The model under review builds one solid part; all positions refer to its coordinate system, in mm. A direction names the side the tool comes from. Coordinates: 2 decimals unless noted, no trailing zeros. Write each loop counter-clockwise with the first axis right and the second up, starting at its lowest first coordinate (ties: lowest second). Pieces come first, ordered by that corner, then holes. Notation, with made-up numbers: (51, -33.5) - (109, -33.5) arc R20 ccw to (109, -17.5) - close; hole circle Ø10 at (28, -27). An arc over 180 degrees is marked (long way). Put each result on its own line as item: value.
Autodesk Inventor part; units mm, degrees
ref_plane "YZ Plane" through (0, 0, 0) normal (1, 0, 0) x (0, 1, 0)
ref_plane "XZ Plane" through (0, 0, 0) normal (0, 1, 0) x (-1, 0, 0)
ref_plane "XY Plane" through (0, 0, 0) normal (0, 0, 1) x (1, 0, 0)
sketch "Sketch1" plane through (0, 0, 0) normal (0, 0, 1) x (1, 0, 0)
  line L0 (0, 0) -> (50.8, 0)
  line L1 (50.8, 0) -> (50.8, 50.8)
  line L2 (50.8, 50.8) -> (0, 50.8)
  line L3 (0, 50.8) -> (0, 0)
  dimension "d0" = 50.8
  dimension "d1" = 50.8
extrude "Extrusion1" add sketch "Sketch1" along normal blind 50.8
sketch "Sketch2" plane through (0, 0, 50.8) normal (0, 0, 1) x (1, 0, 0)
  point P0 (0, 0)
sketch "Sketch3" plane through (0, 0, 50.8) normal (0, 0, 1) x (1, 0, 0)
  circle A0 centre (25.4, 25.4) radius 12.7
  line L0 (0, 50.8) -> (0, 0)
  line L1 (50.8, 50.8) -> (0, 50.8)
  dimension "d4" = 25.4
  dimension "d5" = 25.4
  dimension "d6" = 25.4
extrude "Extrusion2" cut sketch "Sketch3" against normal blind 50.8
sketch "Sketch4" plane through (50.8, 0, 0) normal (1, 0, 0) x (0, 0, -1)
  circle A0 centre (-25.4, 25.4) radius 12.7
  line L0 (-50.8, 0) -> (-50.8, 50.8)
  line L1 (0, 0) -> (0, 50.8)
  line L2 (0, 0) -> (-50.8, 0)
  dimension "d9" = 25.4
  dimension "d10" = 25.4
  dimension "d11" = 25.4
  dimension "d12" = 25.4
extrude "Extrusion3" cut sketch "Sketch4" against normal blind 50.8
chamfer "Chamfer1" distance 3.175 angle 45 12 edges at (25.4, 50.8, 50.8) (0, 50.8, 25.4) (25.4, 50.8, 0) (50.8, 50.8, 25.4) (50.8, 25.4, 50.8) (50.8, 25.4, 0) (50.8, 0, 25.4) (25.4, 0, 0) (25.4, 0, 50.8) (0, 25.4, 50.8) (0, 0, 25.4) (0, 25.4, 0)
fillet "Fillet1" radius 3.175 4 edges at (12.7, 25.4, 50.8) (50.8, 25.4, 38.1) (12.7, 25.4, 0) (0, 25.4, 38.1)
sketch "Sketch5" plane through (3.175, 50.8, 3.175) normal (0, 1, 0) x (1, 0, 0)
  line L0 (22.225, -22.225) -> (9.525, -34.925)
  circle A0 centre (22.225, -22.225) radius 12.7
  point P0 (-3.175, 3.175)
  dimension "d19" = 25.4
extrude "Extrusion4" add sketch "Sketch5" along normal blind 25.4
sketch "Sketch6" plane through (25.4, 76.2, 25.4) normal (0, 1, 0) x (1, 0, 0)
  point P0 (-25.4, 25.4)
fillet "Fillet2" radius 3.175 1 edges at (12.7, 76.2, 25.4)
sketch "Sketch12" plane through (25.4, 76.2, 25.4) normal (0, 1, 0) x (1, 0, 0)
  line L0 (-12.7, 12.7) -> (0, 0)
  circle A0 centre (0, 0) radius 7.3279
  line L1 (0, 7.3279) -> (6.3461, 3.6639)
  line L2 (6.3461, 3.6639) -> (6.3461, -3.6639)
  line L3 (6.3461, -3.6639) -> (0, -7.3279)
  line L4 (0, -7.3279) -> (-6.3461, -3.664)
  line L5 (-6.3461, -3.664) -> (-6.3461, 3.6639)
  line L6 (-6.3461, 3.6639) -> (0, 7.3279)
  point P0 (-25.4, 25.4)
  dimension "d33" = 14.6558
sketch "Sketch13" plane through (25.4, 76.2, 25.4) normal (0, 1, 0) x (1, 0, 0)
  point P0 (-25.4, 25.4)
extrude "Extrusion7" add sketch "Sketch12" along normal blind 9.652 contours L6 L1 L2 L3 L4 L5
chamfer "Chamfer4" distance 1.1906 angle 45 6 edges at (22.2269, 85.852, 30.8959) (28.5731, 85.852, 30.8959) (31.7461, 85.852, 25.4) (28.5731, 85.852, 19.9041) (22.2269, 85.852, 19.9041) (19.0539, 85.852, 25.4)
properties part number "orthographic3"
1. The part is to be moulded in two halves that separate along Y. For faces 6 (the flat face through (20, 41, 0)), 7 (the cylindrical face through (22.65, 13, 39.14)), 8 (the flat face through (48.63, 1.96, 2.22)), say which applies: +Y half, -Y half, draft (parallel to the pull), parting line (faces both ways), or undercut.
Determined:
face 6: draft
face 7: undercut
face 8: -Y half
2. Machinability: for faces 1 (the flat face through (22.18, 80.37, 19.93)), 2 (the flat face through (1.61, 49.235, 25.089)), 3 (the flat face through (31.746, 80, 25)), 4 (the flat face through (22.27, 80.37, 30.92)), 5 (the cylindrical face through (16.04, 61.757, 33.983)), which of the approach directions +Z, -Z, +X, -X, +Y, -Y give a long, thin tool a straight path to every point of the face, cutting with its end or side? Answer none if there is none.
Determined:
face 1: -Z, -X, +Y
face 2: +Z, -Z, -X, +Y
face 3: +Z, -Z, +X, +Y
face 4: +Z, -X, +Y
face 5: +Y
3. Consider section D-D on y = 34. Give the number of separate pieces and of enclosed holes in the cut face, plus the area to 3 significant figures.
Determined:
separate pieces: 4
enclosed holes: 0
area: 988 mm^2
4. Consider section A-A on y = 25.4. State the section outline as (x, z) points (3 decimals), plus the area to 3 significant figures.
Determined:
outline: (0, 3.175) - (3.175, 0) - (9.525, 0) arc R3.175 ccw to (12.7, 3.175) - (12.7, 12.7) - (3.175, 12.7) arc R3.175 ccw to (0, 9.525) - close; (0, 41.275) arc R3.175 ccw to (3.175, 38.1) - (12.7, 38.1) - (12.7, 47.625) arc R3.175 ccw to (9.525, 50.8) - (3.175, 50.8) - (0, 47.625) - close; (38.1, 3.175) arc R3.175 ccw to (41.275, 0) - (47.625, 0) - (50.8, 3.175) - (50.8, 9.525) arc R3.175 ccw to (47.625, 12.7) - (38.1, 12.7) - close; (38.1, 38.1) - (47.625, 38.1) arc R3.175 ccw to (50.8, 41.275) - (50.8, 47.625) - (47.625, 50.8) - (41.275, 50.8) arc R3.175 ccw to (38.1, 47.625) - close
area: 608 mm^2
5. Consider section B-B on z = 7. State the section outline as (x, y) points (3 decimals).
Determined:
outline: (0, 3.175) - (3.175, 0) - (47.625, 0) - (50.8, 3.175) - (50.8, 47.625) - (47.625, 50.8) - (3.175, 50.8) - (0, 47.625) - close; hole circle Ø25.4 at (25.4, 25.4)
6. Consider section C-C on y = 57. State the section outline as (x, z) points, plus the area to 3 significant figures.
Determined:
outline: circle Ø25.4 at (25.4, 25.4)
area: 507 mm^2
7. For pin 1 Ø4 at (x, z) = (28, 41.5) entering from +Y; pin 2 Ø2 at (x, y) = (37.5, 66) entering from -Z; pin 3 Ø5 at (x, y) = (25, 56) entering from +Z, all flat-tipped, find the tip position at first contact; note any pin that passes through.
Determined:
pin 1: stops at y = 50.8
pin 2: stops at z = 19.23
pin 3: stops at z = 38.1
8. To check wall thickness, follow probe 1 along Y at (x, z) = (25, 12); probe 2 along Y at (x, z) = (25.4, 34); probe 3 along X at (y, z) = (25.4, 42.5). State the ranges of each line that lie inside material, in increasing order.
Determined:
probe 1: y = 0 to 12.71, 38.09 to 50.8
probe 2: y = 0 to 12.7, 38.1 to 76.2
probe 3: x = 0 to 12.7, 38.1 to 50.8
